The model under review builds one solid part; all positions refer to its coordinate system, in mm. Coordinates: 2 decimals unless noted, no trailing zeros. Order: outer loops, then holes, each group sorted by start corner. A loop starts at its lowest first (then second) coordinate and runs counter-clockwise, first axis right, second up. Notation, with made-up numbers: (85.25, 48) -> (114.25, 48) arc R28 cw to (114.25, 66) -> close; hole circle Ø11 at (80, -28). An arc over 180 degrees is marked (long way). Put each result on its own line as item: value.
from build123d import *

# Parameters (mm, degrees)
SKETCH_W      = 188
SKETCH_H      = 188
PAD_DEPTH     = 4
SKETCH001_R   = 1.625
POCKET_DEPTH  = 4.001
FILLET_R      = 3
SKETCH003_W   = 150
SKETCH003_H   = 8
SKETCH003_W_2 = 8
SKETCH003_H_2 = 150
PAD001_DEPTH  = 2
FILLET001_R   = 1


with BuildPart() as part:
    # Sketch → Pad (new body)
    with BuildSketch(Plane.XY):
        Rectangle(SKETCH_W, SKETCH_H)
    extrude(amount=PAD_DEPTH)

    # Sketch001 (on Face6 of Pad) → Pocket (cut, through all)
    with BuildSketch(Plane.XY.offset(4)):
        with Locations((-89, 89)):
            Circle(SKETCH001_R)
        with Locations((89, 89)):
            Circle(SKETCH001_R)
        with Locations((89, -89)):
            Circle(SKETCH001_R)
        with Locations((-89, -89)):
            Circle(SKETCH001_R)
    extrude(amount=-POCKET_DEPTH, mode=Mode.SUBTRACT)

    # Fillet
    fillet_edges = [part.edges().sort_by_distance(p)[0] for p in [
        (-94, 94, 2),
        (94, 94, 2),
        (-94, -94, 2),
        (94, -94, 2),
    ]]
    fillet(fillet_edges, radius=FILLET_R)

    # Sketch003 (on Face5 of Fillet) → Pad001 (join)
    with BuildSketch(Plane.XY.offset(4)):
        with Locations((0, -83.5)):
            Rectangle(SKETCH003_W, SKETCH003_H)
        with Locations((0, 83.5)):
            Rectangle(SKETCH003_W, SKETCH003_H)
        with Locations((-85.5, 0)):
            Rectangle(SKETCH003_W_2, SKETCH003_H_2)
        with Locations((85.5, 0)):
            Rectangle(SKETCH003_W_2, SKETCH003_H_2)
    extrude(amount=PAD001_DEPTH)

    # Fillet001
    fillet001_edges = [part.edges().sort_by_distance(p)[0] for p in [
        (-85.5, 75, 6),
        (-81.5, 0, 6),
        (-85.5, -75, 6),
        (-89.5, 0, 6),
        (0, -79.5, 6),
        (75, -83.5, 6),
        (0, -87.5, 6),
        (-75, -83.5, 6),
        (85.5, 75, 6),
        (89.5, 0, 6),
        (85.5, -75, 6),
        (81.5, 0, 6),
        (0, 87.5, 6),
        (75, 83.5, 6),
        (0, 79.5, 6),
        (-75, 83.5, 6),
    ]]
    fillet(fillet001_edges, radius=FILLET001_R)


solid = part.part
Item 1: Consider section A-A on x = 67.5. Write out the cut boundary in (y, z), and give its area (3 significant figures).
Answers below:
outline: (-94, 0) -> (94, 0) -> (94, 4) -> (87.5, 4) -> (87.5, 5) arc R1 ccw to (86.5, 6) -> (80.5, 6) arc R1 ccw to (79.5, 5) -> (79.5, 4) -> (-79.5, 4) -> (-79.5, 5) arc R1 ccw to (-80.5, 6) -> (-86.5, 6) arc R1 ccw to (-87.5, 5) -> (-87.5, 4) -> (-94, 4) -> close
area: 783 mm^2
Item 2: Consider section B-B on y = 26. Write out the cut boundary in (x, z), and give its area (3 significant figures).
Answers below:
outline: (-94, 0) -> (94, 0) -> (94, 4) -> (89.5, 4) -> (89.5, 5) arc R1 ccw to (88.5, 6) -> (82.5, 6) arc R1 ccw to (81.5, 5) -> (81.5, 4) -> (-81.5, 4) -> (-81.5, 5) arc R1 ccw to (-82.5, 6) -> (-88.5, 6) arc R1 ccw to (-89.5, 5) -> (-89.5, 4) -> (-94, 4) -> close
area: 783 mm^2
Item 3: For pin 1 Ø3 at (x, y) = (-89, -89) entering from +Z; pin 2 Ø0.5 at (y, z) = (30, 4.5) entering from -X; pin 3 Ø0.5 at (y, z) = (-85, 4.5) entering from -X; pin 4 Ø0.5 at (x, z) = (32, 4.5) entering from -Y, all flat-tipped, find the tip position at first contact; note any pin that passes through.
Answers below:
pin 1: through
pin 2: x = -89.5
pin 3: x = -75
pin 4: y = -87.5
Item 4: For line 1 (X direction, y = -89, z = 0.9) (3 decimals); line 2 (Y direction, x = 30.5, z = 5.2), list the stretches that pass through material, from the lowest coordinate up. Write a range as from..to.
Answers below:
line 1: -94..-90.625, -87.375..87.375, 90.625..94
line 2: -87.48..-79.52, 79.52..87.48
Item 5: Consider section C-C on x = -78.5. Write out the cut boundary in (y, z).
Answers below:
outline: (-94, 0) -> (94, 0) -> (94, 4) -> (-94, 4) -> close
Item 6: Mouldability with a two-part tool opening along Y and no side actions: class faces 1 (the flat face through (-1, 1, 4)), 2 (the flat face through (-1, 84, 6)), 3 (the flat face through (-1, 94, 2)), 4 (the flat face through (-1, -94, 2)) as +Y half, -Y half, draft (parallel to the pull), parting line (faces both ways), or undercut.
Answers below:
face 1: undercut
face 2: draft
face 3: +Y half
face 4: -Y half
